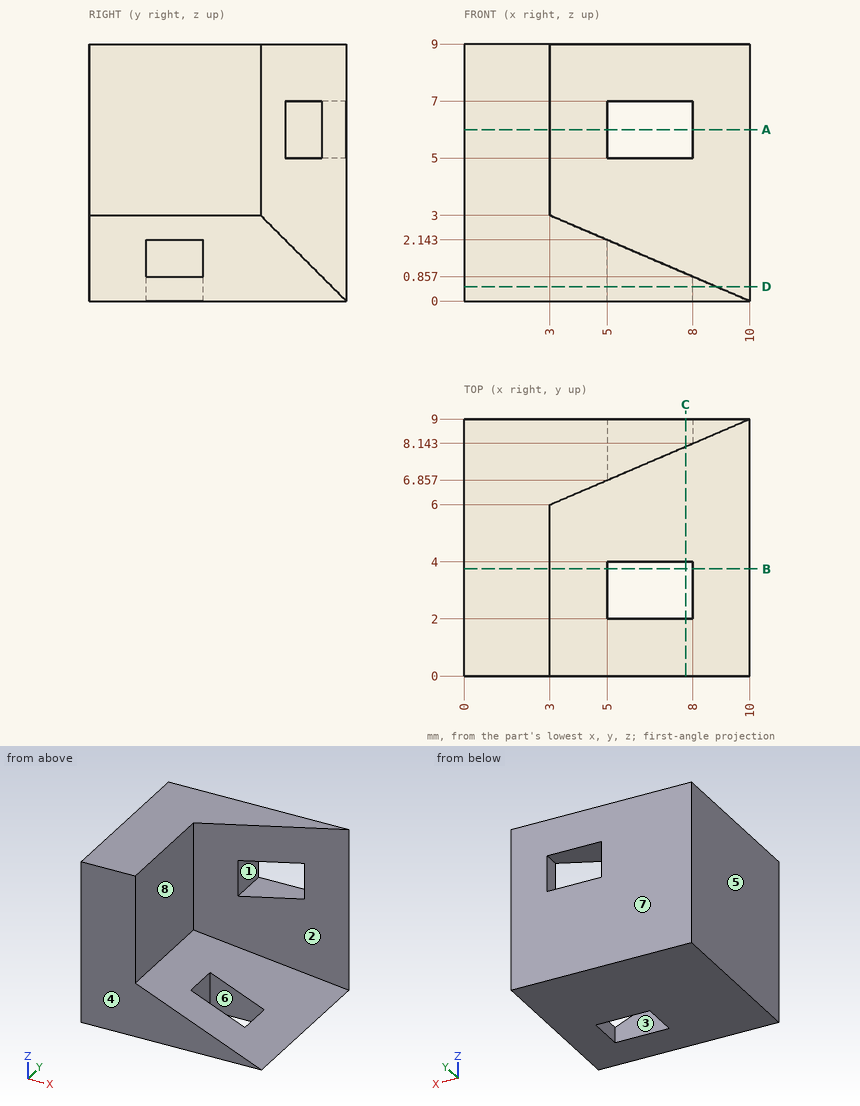
Print and shaded views of the part. All mm, measured from the part's lowest x, y and z. A direction names the side the tool comes from. Coordinates: 2 decimals unless noted, no trailing zeros. Order: outer loops, then holes, each group sorted by start corner. A loop starts at its lowest first (then second) coordinate and runs counter-clockwise, first axis right, second up. Notation, with made-up numbers: (55.5, -20.75) - (86.5, -20.75) arc R29 ccw to (86.5, 8.25) - close; hole circle Ø8 at (-4.75, 48.5). An arc over 180 degrees is marked (long way). Put each result on its own line as item: value.
1. Pull direction X, two halves, no side cores. Call the marked faces 6, 7 and 8: pulls with the +X half, pulls with the -X half, needs draft (parallel to the pull), parting line crosses it, or undercut.
Answer sheet:
face 6: undercut
face 7: needs draft
face 8: pulls with the +X half
2. Probe line 1 along Z through (x, y) = (5.25, 7); line 2 along Z through (x, y) = (5, 5.75); line 3 along X through (y, z) = (5.5, 5.5). List the from-to ranges inside material, lowest first. Write a range as [from, to].
Answer sheet:
line 1: z = [0, 5], [7, 9]
line 2: z = [0, 2.14]
line 3: x = [0, 3]
3. Saw through at D-D (z = 0.5). Write the cut outline in (x, y).
Answer sheet:
outline: (0, 0) - (8.83, 0) - (8.83, 8.5) - (10, 9) - (0, 9) - close; hole (5, 2) - (8, 2) - (8, 4) - (5, 4) - close
4. Tool access for the marked faces 1, 2, 3, 4 and 5: list every direction of +Z, -Z, +X, -X, +Y, -Y with a clear straight run to the whole face (end or side of a thin tool).
Answer sheet:
face 1: +Y, -Y
face 2: +Z, +X, -Y
face 3: +Z, -Z
face 4: +Z, -Z, +X, -X, -Y
face 5: +Z, -Z, -X, +Y, -Y
5. Saw through at C-C (x = 7.75). Write the cut outline in (y, z), and give its area (3 significant figures).
Answer sheet:
outline: (0, 0) - (2, 0) - (2, 0.96) - (0, 0.96) - close; (4, 0) - (9, 0) - (9, 5) - (8.04, 5) - (8.04, 0.96) - (4, 0.96) - close; (8.04, 7) - (9, 7) - (9, 9) - (8.04, 9) - close
area: 12.6 mm^2
6. Saw through at A-A (z = 6). Write the cut outline in (x, y).
Answer sheet:
outline: (0, 0) - (3, 0) - (3, 6) - (5, 6.86) - (5, 9) - (0, 9) - close; (8, 8.14) - (10, 9) - (8, 9) - close
7. Saw through at B-B (y = 3.75). Write the cut outline in (x, z).
Answer sheet:
outline: (0, 0) - (5, 0) - (5, 2.14) - (3, 3) - (3, 9) - (0, 9) - close; (8, 0) - (10, 0) - (8, 0.86) - close
8. Drop flat-ended pins along their axis: P1, Ø2.5, axis at x = 6.5, y = 7.5, coming from the -Z side; P2, Ø0.6, axis at y = 8, z = 6, coming from the +X side; P3, Ø3, axis at y = 4, z = 5.5, coming from the +X side; P4, Ø1.6, axis at y = 3.5, z = 1, coming from the +X side. Give the stop position or say it passes through.
Answer sheet:
P1: stops at z = 0
P2: stops at x = 8.37
P3: stops at x = 3
P4: stops at x = 9.53
